Can you work these out from the model? Positions are in its coordinate system, mm. Give positions to 0.01 mm unless a question says otherwise; leave off trailing zeros. Write each loop counter-clockwise with the first axis right and the second up, starting at its lowest first coordinate (ties: lowest second). Pieces come first, ordered by that corner, then holes.
```python
from build123d import *

# Parameters (mm, degrees)
SKETCH6_R           = 19.15
BOSS_EXTRUDE3_DEPTH = 75
SKETCH9_R           = 3.7
CUT_EXTRUDE2_DEPTH  = 5.15


with BuildPart() as part:
    # Sketch6 → Boss-Extrude3 (new body)
    with BuildSketch(Plane.XY):
        Circle(SKETCH6_R)
    extrude(amount=BOSS_EXTRUDE3_DEPTH)

    # Sketch9 → Cut-Extrude2 (cut)
    with BuildSketch(Plane.XY.offset(75)):
        Circle(SKETCH9_R)
        with Locations((-15, 0)):
            Circle(SKETCH9_R)
        with Locations((15, 0)):
            Circle(SKETCH9_R)
    extrude(amount=-CUT_EXTRUDE2_DEPTH, mode=Mode.SUBTRACT)


solid = part.part
```
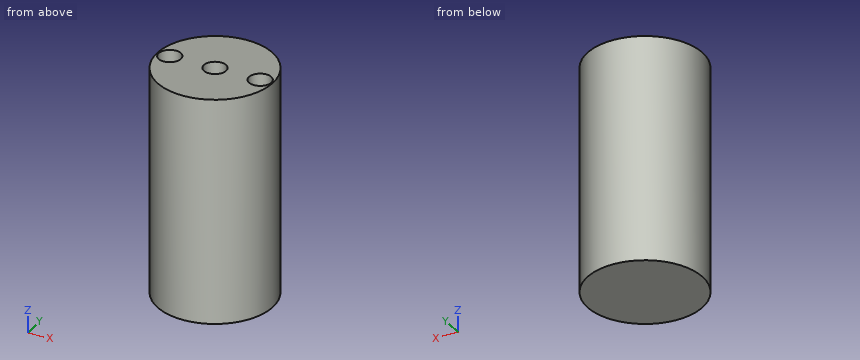
1) Suppose I cut it at D-D on y = -15. Write out the boundary of the cut face in (x, z), plus the area to 3 significant figures.
Values follow:
outline: (-11.9, 0) - (11.9, 0) - (11.9, 75) - (-11.9, 75) - close
area: 1,790 mm2
2) Please list where these lines run through material, in increasing order: L1, parallel to Y at x = 0, z = 72.1; L2, parallel to Y at x = 0, z = 37; L3, parallel to Y at x = 11.5, z = 60.
Values follow:
L1: y = -19.15 to -3.7, 3.7 to 19.15
L2: y = -19.15 to 19.15
L3: y = -15.31 to 15.31
3) For pin 1 Ø6 at (x, z) = (3, 15) entering from +Y; pin 2 Ø12 at (x, y) = (-11.5, 4.5) entering from -Z; pin 3 Ø4.5 at (x, y) = (0, 0) entering from +Z; pin 4 Ø10 at (y, z) = (-13.5, 23.5) entering from -X, each with a flat end and sliding along its axis, tell me the tip position at first contact or that it passes through.
Values follow:
pin 1: stops at y = 19.15
pin 2: stops at z = 0
pin 3: stops at z = 69.85
pin 4: stops at x = -17.16
4) Suppose I cut it at A-A on y = 0. Write out the boundary of the cut face in (x, z).
Values follow:
outline: (-19.15, 0) - (19.15, 0) - (19.15, 75) - (18.7, 75) - (18.7, 69.85) - (11.3, 69.85) - (11.3, 75) - (3.7, 75) - (3.7, 69.85) - (-3.7, 69.85) - (-3.7, 75) - (-11.3, 75) - (-11.3, 69.85) - (-18.7, 69.85) - (-18.7, 75) - (-19.15, 75) - close
5) Suppose I cut it at B-B on z = 54. Write out the boundary of the cut face in (x, y).
Values follow:
outline: circle Ø38.3 at (0, 0)
6) Suppose I cut it at C-C on x = 15. Write out the boundary of the cut face in (y, z).
Values follow:
outline: (-11.9, 0) - (11.9, 0) - (11.9, 75) - (3.7, 75) - (3.7, 69.85) - (-3.7, 69.85) - (-3.7, 75) - (-11.9, 75) - close
